Read the model definition and answer for the solid it produces. Units are mm, in the model's axes. A direction names the side the tool comes from. Coordinates: 2 decimals unless noted, no trailing zeros. Loops run counter-clockwise (first coordinate to the right, second up) from the corner with the lowest first, then second, coordinate; pieces in that order, holes last. Notation, with made-up numbers: (68.5, 27.25) -> (89.5, 27.25) arc R26 cw to (89.5, 54.25) -> close; hole circle Ø11 at (8.5, 18). An arc over 180 degrees is marked (long way). Answer as a JSON object with one key per item and string values. Group by question number.
1) Section A-A, the plane z = 37.5 is taken. Give the vertices of the cut face in (x, y), plus the area to 3 significant figures.
2) Determine the mould class of faces 4 (the face through (21, -17, 16)), 5 (the face through (-11, 0, 3)), 6 (the face through (22.5, 0, 25)), 7 (the face through (21.021, -21.17, 36.733)) for opening direction Z: released by +Z, released by -Z, zero draft, split by the parting line, or undercut.
3) Section C-C, the plane y = 0 is taken. Give the vertices of the cut face in (x, z).
4) Which of the six approach directions +Z, -Z, +X, -X, +Y, -Y give full straight-line access (tool end or side, diameter ignored) to faces 1 (the face through (-2, 5, 6)), 2 (the face through (8.1, -1.3, 3)), 3 (the face through (5, 10, 4))?
5) Section B-B, the plane y = 21.41 is taken. Give the vertices of the cut face in (x, z), plus the area to 3 significant figures.
6) Flat-ended cylindrical pins translate along their axes: P1, Ø8, axis at x = -18, z = 4.5, coming from the -Y side; P2, Ø1.8, axis at x = -14.5, y = 1.5, coming from the +Z side; P3, Ø8, axis at x = 3, z = 8, coming from the +Y side. Find the tip coordinate at first contact, or state that the pin passes through.
7) Consider probe 1 along Z at (x, y) = (20, 21); probe 2 along X at (y, z) = (8, 10.5); probe 3 along Z at (x, y) = (-15.5, -7.5). Determine where each line is inside the solid, lowest interval first. Write a range as [from, to].
8) Section D-D, the plane x = -17.5 is taken. Give the vertices of the cut face in (y, z), plus the area to 3 significant figures.
from build123d import *

# Parameters (mm, degrees)
CROQUIS1_W              = 45
CROQUIS1_H              = 20
SALIENTE_EXTRUIR1_DEPTH = 6
CROQUIS2_W              = 3
CROQUIS2_H              = 20
SALIENTE_EXTRUIR2_DEPTH = 10
SALIENTE_EXTRUIR3_DEPTH = 25
CROQUIS4_R              = 0.8
CROQUIS4_W              = 11
CROQUIS4_H              = 11
CORTAR_EXTRUIR1_DEPTH   = 66.810333535
CROQUIS5_R              = 0.998921469
CROQUIS5_R_2            = 1
CORTAR_EXTRUIR2_DEPTH   = 49.541219597
CORTAR_EXTRUIR3_DEPTH   = 3
CROQUIS7_R              = 3.5
CORTAR_EXTRUIR4_DEPTH   = 49.541219597


with BuildPart() as part:
    # Croquis1 → Saliente-Extruir1 (new body)
    with BuildSketch(Plane.XY):
        Rectangle(CROQUIS1_W, CROQUIS1_H)
    extrude(amount=SALIENTE_EXTRUIR1_DEPTH)

    # Croquis2 → Saliente-Extruir2 (add)
    with BuildSketch(Plane.XY.offset(6)):
        with Locations((21, 0)):
            Rectangle(CROQUIS2_W, CROQUIS2_H)
    extrude(amount=SALIENTE_EXTRUIR2_DEPTH)

    # Croquis3 → Saliente-Extruir3 (add)
    with BuildSketch(Plane.XY.offset(16)):
        Polygon((19.5, 0), (19.5, 25), (22.5, 25), (22.5, -25), (19.5, -25), align=None)
    extrude(amount=SALIENTE_EXTRUIR3_DEPTH)

    # Croquis4 → Cortar-Extruir1 (cut, through all)
    with BuildSketch(Plane(origin=(22.5, 0, 0), x_dir=(0, 0, -1), z_dir=(1, 0, 0))):
        with Locations((-19.756259271, -21.41)):
            Circle(CROQUIS4_R)
        with Locations((-37.496259271, -21.41)):
            Circle(CROQUIS4_R)
        with Locations((-19.756259271, 21.41)):
            Circle(CROQUIS4_R)
        with Locations((-37.496259271, 21.41)):
            Circle(CROQUIS4_R)
        with Locations((-41, 0)):
            Rectangle(CROQUIS4_W, CROQUIS4_H)
    extrude(amount=-CORTAR_EXTRUIR1_DEPTH, mode=Mode.SUBTRACT)

    # Croquis5 → Cortar-Extruir2 (cut, through all)
    with BuildSketch(Plane.XY.offset(6)):
        with Locations((-20.857855881, 0)):
            Circle(CROQUIS5_R)
        with Locations((7.642144119, 0)):
            Circle(CROQUIS5_R_2)
    extrude(amount=-CORTAR_EXTRUIR2_DEPTH, mode=Mode.SUBTRACT)

    # Croquis6 → Cortar-Extruir3 (cut)
    with BuildSketch(Plane.XY.offset(6)):
        with BuildLine():
            Line((-16.706350445, 2.011408213), (-3.374218766, 2.960859602))
            Line((-3.374218766, 2.960859602), (0.362949608, 2.958054567))
            Line((0.362949608, 2.958054567), (13.588372541, 1.996246225))
            ThreePointArc((13.588372541, 1.996246225), (15.702474132, -0.012917688), (13.585358857, -2.018905744))
            Line((13.585358857, -2.018905744), (0.358507003, -2.960859602))
            Line((0.358507003, -2.960859602), (-3.37866137, -2.958054567))
            Line((-3.37866137, -2.958054567), (-16.709352754, -1.988590661))
            ThreePointArc((-16.709352754, -1.988590661), (-18.707851036, 0.012909931), (-16.706350445, 2.011408213))
        make_face()
    extrude(amount=-CORTAR_EXTRUIR3_DEPTH, mode=Mode.SUBTRACT)

    # Croquis7 → Cortar-Extruir4 (cut, through all)
    with BuildSketch(Plane.XY.offset(6)):
        with Locations((-1.507855881, 0)):
            Circle(CROQUIS7_R)
    extrude(amount=-CORTAR_EXTRUIR4_DEPTH, mode=Mode.SUBTRACT)


solid = part.part
Determined:
{
 "1": {"outline": "(19.5, -25) -> (22.5, -25) -> (22.5, -22.21) -> (19.5, -22.21) -> close; (19.5, -20.61) -> (22.5, -20.61) -> (22.5, -5.5) -> (19.5, -5.5) -> close; (19.5, 5.5) -> (22.5, 5.5) -> (22.5, 20.61) -> (19.5, 20.61) -> close; (19.5, 22.21) -> (22.5, 22.21) -> (22.5, 25) -> (19.5, 25) -> close", "area": "107 mm²"},
 "2": {"face 4": "released by -Z", "face 5": "released by +Z", "face 6": "zero draft", "face 7": "undercut"},
 "3": {"outline": "(-22.5, 0) -> (-21.86, 0) -> (-21.86, 6) -> (-22.5, 6) -> close; (-19.86, 0) -> (-5.01, 0) -> (-5.01, 3) -> (-18.71, 3) -> (-18.71, 6) -> (-19.86, 6) -> close; (1.99, 0) -> (6.64, 0) -> (6.64, 3) -> (1.99, 3) -> close; (8.64, 0) -> (22.5, 0) -> (22.5, 35.5) -> (19.5, 35.5) -> (19.5, 6) -> (15.7, 6) -> (15.7, 3) -> (8.64, 3) -> close"},
 "4": {"face 1": "+Z, -X, +Y, -Y", "face 2": "+Z", "face 3": "-Z, +X, -X, +Y"},
 "5": {"outline": "(19.5, 16) -> (22.5, 16) -> (22.5, 18.96) -> (19.5, 18.96) -> close; (19.5, 20.56) -> (22.5, 20.56) -> (22.5, 36.7) -> (19.5, 36.7) -> close; (19.5, 38.3) -> (22.5, 38.3) -> (22.5, 41) -> (19.5, 41) -> close", "area": "65.4 mm²"},
 "6": {"P1": "y = -10", "P2": "z = 6", "P3": "y = 10"},
 "7": {"probe 1": "[16, 19.07], [20.44, 36.81], [38.18, 41]", "probe 2": "[19.5, 22.5]", "probe 3": "[0, 6]"},
 "8": {"outline": "(-10, 0) -> (10, 0) -> (10, 6) -> (1.85, 6) -> (1.85, 3) -> (-1.83, 3) -> (-1.83, 6) -> (-10, 6) -> close", "area": "109 mm²"}
}
